Could you check a few things on this model? Use its own coordinates, in mm. Face numbers are marked on the shaded views. A direction names the side the tool comes from. Coordinates: 2 decimals unless noted, no trailing zeros. Loops run counter-clockwise (first coordinate to the right, second up) from the corner with the lowest first, then second, coordinate; pieces in that order, holes last. Notation, with made-up numbers: (45, 42) - (69, 42) arc R35 ccw to (69, 77) - close; hole circle Ø8 at (51, 40.25). An arc over 180 degrees is marked (long way). One line per item, written item: value. Start each with the question number.
(1) If we section it at C-C on y = 4.8: Write out the boundary of the cut face in (x, z).
(2) On a 3-axis mill with a long thin cutter (end or side, diameter ignored), from which of +Z, -Z, +X, -X, +Y, -Y can I reach the whole of each face in a straight line? I mean the marked faces 4 and 5. Say none if no direction works.
(3) If we mould it in two halves opening along X, with no side actions, what happens to the marked faces 1, 2 and 3? For each: pulls with the +X half, pulls with the -X half, needs draft (parallel to the pull), parting line crosses it, or undercut.
(4) If we section it at D-D on z = 16.75: Write out the boundary of the cut face in (x, y).
(5) If I drill on line 1 along Y through (x, z) = (4.8, 17.75); line 2 along X through (y, z) = (52, 14.5); line 3 along X through (y, z) = (52.5, 17.75), over which ranges is the centre line in solid material (lowest first)? Write a range as from..to.
(6) I'm going to push a flat-ended pin straight in: P1, Ø1.5, axis at x = 32, z = 4.5, coming from the -Y side. Where does the tip first touch, or does it pass through?
(7) If we section it at A-A on x = 4.8: Write out the boundary of the cut face in (y, z).
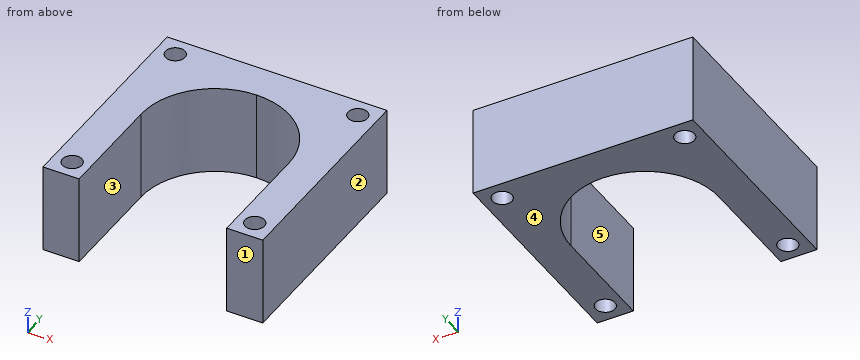
```python
from build123d import *

# Parameters (mm, degrees)
F0_W     = 56.6
F0_H     = 56.6
F1_DEPTH = 23
F3_DEPTH = 23
F5_D     = 5


with BuildPart() as f1:
    # F0 (on Top) → F1 (new body)
    with BuildSketch(Plane.XY):
        with Locations((28.3, 28.3)):
            Rectangle(F0_W, F0_H)
    extrude(amount=F1_DEPTH)

    # F2 (on face) → F3 (cut, through all)
    with BuildSketch(Plane.XY.offset(23)):
        with BuildLine():
            Line((28.3, 28.3), (47.3, 28.3))
            ThreePointArc((47.3, 28.3), (41.7350288425, 41.7350288425), (28.3, 47.3))
            Line((28.3, 47.3), (28.3, 28.3))
        make_face()
        with BuildLine():
            Line((47.3, 0), (47.3, 28.3))
            ThreePointArc((47.3, 28.3), (41.7350288425, 14.8649711575), (28.3, 9.3))
            Line((28.3, 9.3), (28.3, 0))
            Line((28.3, 0), (47.3, 0))
        make_face()
        with BuildLine():
            ThreePointArc((28.3, 9.3), (41.7350288425, 14.8649711575), (47.3, 28.3))
            Line((47.3, 28.3), (28.3, 28.3))
            Line((28.3, 28.3), (28.3, 9.3))
        make_face()
        with BuildLine():
            Line((28.3, 28.3), (28.3, 47.3))
            ThreePointArc((28.3, 47.3), (14.8649711575, 41.7350288425), (9.3, 28.3))
            Line((9.3, 28.3), (28.3, 28.3))
        make_face()
        with BuildLine():
            Line((28.3, 0), (28.3, 9.3))
            ThreePointArc((28.3, 9.3), (14.8649711575, 14.8649711575), (9.3, 28.3))
            Line((9.3, 28.3), (9.3, 0))
            Line((9.3, 0), (28.3, 0))
        make_face()
        with BuildLine():
            ThreePointArc((9.3, 28.3), (14.8649711575, 14.8649711575), (28.3, 9.3))
            Line((28.3, 9.3), (28.3, 28.3))
            Line((28.3, 28.3), (9.3, 28.3))
        make_face()
    extrude(amount=-F3_DEPTH, mode=Mode.SUBTRACT)

    # F5 (through all)
    with Locations(Plane.XY.offset(23)):
        with Locations((4.8, 51.8), (51.8, 51.8), (51.8, 4.8), (4.8, 4.8)):
            Hole(F5_D / 2)


solid = f1.part
```
Values:
1. outline: (0, 0) - (2.3, 0) - (2.3, 23) - (0, 23) - close; (7.3, 0) - (9.3, 0) - (9.3, 23) - (7.3, 23) - close; (47.3, 0) - (49.3, 0) - (49.3, 23) - (47.3, 23) - close; (54.3, 0) - (56.6, 0) - (56.6, 23) - (54.3, 23) - close
2. face 4: -Z, +X, -X, +Y, -Y
2. face 5: +Z, -Z, -Y
3. face 1: needs draft
3. face 2: pulls with the +X half
3. face 3: undercut
4. outline: (0, 0) - (9.3, 0) - (9.3, 28.3) arc R19 cw to (47.3, 28.3) - (47.3, 0) - (56.6, 0) - (56.6, 56.6) - (0, 56.6) - close; hole circle Ø5 at (4.8, 4.8); hole circle Ø5 at (4.8, 51.8); hole circle Ø5 at (51.8, 4.8); hole circle Ø5 at (51.8, 51.8)
5. line 1: y = 0..2.3, 7.3..49.3, 54.3..56.6
5. line 2: x = 0..2.31, 7.29..49.31, 54.29..56.6
5. line 3: x = 0..2.4, 7.2..49.4, 54.2..56.6
6. P1: stops at y = 46.77
7. outline: (0, 0) - (2.3, 0) - (2.3, 23) - (0, 23) - close; (7.3, 0) - (49.3, 0) - (49.3, 23) - (7.3, 23) - close; (54.3, 0) - (56.6, 0) - (56.6, 23) - (54.3, 23) - close
